Could you check a few things on this model? Use its own coordinates, in mm. A direction names the side the tool comes from. Coordinates: 2 decimals unless noted, no trailing zeros. Order: outer loops, then holes, each group sorted by start corner. A loop starts at its lowest first (then second) coordinate and runs counter-clockwise, first axis right, second up. Notation, with made-up numbers: M -8,87 L 43,87 A14 cw 43,92 Z; hole C 60.5,78.25 d9. An arc over 180 degrees is marked long. One line per question, with ' | ' between items. Start each with the question number.
from build123d import *

# Parameters (mm, degrees)
F1_DEPTH      = 25.4
F2_W          = 25.4
F2_H          = 15.875
F3_DEPTH      = 12.701
F3_DEPTH_BACK = 76.201
F5_DEPTH      = 9.525
F6_R          = 3.683
F7_DEPTH      = 82.551
F8_W          = 25.4
F8_H          = 12.7
F9_DEPTH      = 76.201
F10_R         = 3.683
F11_DEPTH     = 12.701
F12_R         = 8.89
F13_DEPTH     = 7.62


with BuildPart() as f1:
    # F0 (on Front) → F1 (new body, symmetric)
    with BuildSketch(Plane.XZ):
        Polygon((76.2, 0), (0, 0), (0, 63.5), (50.8, 63.5), (50.8, 73.025), (0, 82.55), (-12.7, 82.55), (-12.7, -82.55), (0, -82.55), (0, -31.75), (76.2, -19.05), align=None)
    extrude(amount=F1_DEPTH, both=True)

    # F2 (on Right) → F3 (cut, two sides)
    with BuildSketch(Plane.YZ) as f3_sk:
        with Locations((0, 74.6125)):
            Rectangle(F2_W, F2_H)
    extrude(amount=-F3_DEPTH, mode=Mode.SUBTRACT)
    extrude(f3_sk.sketch, amount=F3_DEPTH_BACK, mode=Mode.SUBTRACT)

    # F4 (on Top) → F5 (cut)
    with BuildSketch(Plane.XY):
        Polygon((19.304, -3.8128211777), (19.304, 3.8128211777), (12.7, 7.6256423555), (6.096, 3.8128211777), (6.096, -3.8128211777), (12.7, -7.6256423555), align=None)
        Polygon((70.1092849155, 3.8036527495), (63.5105825496, 7.6256350124), (56.901297634, 3.821982263), (56.8907150845, -3.8036527495), (63.4894174504, -7.6256350124), (70.098702366, -3.821982263), align=None)
    extrude(amount=-F5_DEPTH, mode=Mode.SUBTRACT)

    # F6 (on Top) → F7 (cut, through all)
    with BuildSketch(Plane.XY):
        with Locations((12.7, 0)):
            Circle(F6_R)
        with Locations((63.5, 0)):
            Circle(F6_R)
    extrude(amount=-F7_DEPTH, mode=Mode.SUBTRACT)

    # F8 (on Right) → F9 (cut, through all)
    with BuildSketch(Plane.YZ):
        with Locations((0, -25.4)):
            Rectangle(F8_W, F8_H)
    extrude(amount=F9_DEPTH, mode=Mode.SUBTRACT)

    # F10 (on Right) → F11 (cut, through all)
    with BuildSketch(Plane.YZ):
        with Locations((-12.7, -44.45)):
            Circle(F10_R)
        with Locations((12.7, -44.45)):
            Circle(F10_R)
        with Locations((-12.7, -69.85)):
            Circle(F10_R)
        with Locations((12.7, -69.85)):
            Circle(F10_R)
        with Locations((-12.7, 19.05)):
            Circle(F10_R)
        with Locations((12.7, 19.05)):
            Circle(F10_R)
        with Locations((-12.7, 44.45)):
            Circle(F10_R)
        with Locations((12.7, 44.45)):
            Circle(F10_R)
    extrude(amount=-F11_DEPTH, mode=Mode.SUBTRACT)

    # F12 (on Right) → F13 (cut)
    with BuildSketch(Plane.YZ):
        with Locations((-12.7, 44.45)):
            Circle(F12_R)
        with Locations((12.7, 44.45)):
            Circle(F12_R)
        with Locations((-12.7, 19.05)):
            Circle(F12_R)
        with Locations((12.7, 19.05)):
            Circle(F12_R)
    extrude(amount=-F13_DEPTH, mode=Mode.SUBTRACT)


solid = f1.part
(1) Imagine slicing it at B-B, the plane z = 44.45. Write out the boundary of the cut face in (x, y).
(2) Imagine slicing it at A-A, the plane z = -2.5. Write out the boundary of the cut face in (x, y), plus the area to 3 significant figures.
(3) Imagine slicing it at D-D, the plane y = 0. Write out the boundary of the cut face in (x, z) (3 decimals).
(4) We'd pull the mould along Z, two halves only. Please class faces 1 (the flat face through (37.57, -19.14, -25.49)), 2 (the flat face through (-6, -19, 82.55)), 3 (the flat face through (76.2, 0, -10)), 4 (the cylindrical face through (-10.124, 11.902, 15.455)): +Z half, -Z half, draft (parallel to the pull), parting line (faces both ways), or undercut.
(5) On a 3-axis mill with a long thin cutter (end or side, diameter ignored), from which of +Z, -Z, +X, -X, +Y, -Y can I reach the whole of each face in a straight line? I mean faces 5 (the flat face through (12, 12.7, 73)), 6 (the flat face through (0, 0, 31)), 7 (the cylindrical face through (-3.76, -4.22, 47.12)), 8 (the flat face through (66.75, -5.75, -4.7)). Say none if no direction works.
(6) If I drill on line 1 along Y through (x, z) = (-10, 19); line 2 along Z through (x, y) = (-10, -12) (3 decimals); line 3 along Y through (x, z) = (-5, 24.5), over which ranges is the centre line in solid material (lowest first)? Write a range as from..to.
(7) Imagine slicing it at C-C, the plane x = 28. Write out the boundary of the cut face in (y, z) (3 decimals), plus the area to 3 significant figures.
(8) For P1, Ø6.5, axis at x = 12.5, y = -2.5, coming from the +Z side (3 decimals); P2, Ø20.5, axis at x = 13, y = 5.5, coming from the +Z side; P3, Ø3, axis at x = 64, y = -13.5, coming from the -Z side, each with a flat end and sliding along its axis, tell me the tip position at first contact or that it passes through.
Answers:
1) outline: M -12.7,-25.4 L 0,-25.4 L 0,-21.59 L -7.62,-21.59 L -7.62,-16.38 L -12.7,-16.38 Z; M -12.7,-9.02 L -7.62,-9.02 L -7.62,-3.81 L 0,-3.81 L 0,3.81 L -7.62,3.81 L -7.62,9.02 L -12.7,9.02 Z; M -12.7,16.38 L -7.62,16.38 L -7.62,21.59 L 0,21.59 L 0,25.4 L -12.7,25.4 Z
2) outline: M -12.7,-25.4 L 76.2,-25.4 L 76.2,25.4 L -12.7,25.4 Z; hole M 6.1,-3.81 L 12.7,-7.63 L 19.3,-3.81 L 19.3,3.81 L 12.7,7.63 L 6.1,3.81 Z; hole M 56.89,-3.8 L 63.49,-7.63 L 70.1,-3.82 L 70.11,3.8 L 63.51,7.63 L 56.9,3.82 Z | area: 4,210 mm²
3) outline: M -12.7,-82.55 L 0,-82.55 L 0,-19.05 L 9.017,-19.05 L 9.017,-9.525 L 6.096,-9.525 L 6.096,0 L 0,0 L 0,63.5 L 50.8,63.5 L 50.8,66.675 L -12.7,66.675 Z; M 16.383,-19.05 L 59.817,-19.05 L 59.817,-9.525 L 56.896,-9.525 L 56.896,0 L 19.304,0 L 19.304,-9.525 L 16.383,-9.525 Z; M 67.183,-19.05 L 76.2,-19.05 L 76.2,0 L 70.104,0 L 70.104,-9.525 L 67.183,-9.525 Z
4) face 1: -Z half | face 2: +Z half | face 3: draft | face 4: undercut
5) face 5: +Z, +X, -X | face 6: +X, +Y, -Y | face 7: +X | face 8: +Z
6) line 1: -25.4..-16.38, -9.02..9.02, 16.38..25.4 | line 2: -82.55..-73.466, -66.234..-48.066, -40.834..15.434, 22.666..40.834, 48.066..66.675 | line 3: -25.4..-19.72, -5.68..5.68, 19.72..25.4
7) outline: M -25.4,-27.083 L -12.7,-27.083 L -12.7,-19.05 L 12.7,-19.05 L 12.7,-27.083 L 25.4,-27.083 L 25.4,0 L -25.4,0 Z; M -25.4,63.5 L 25.4,63.5 L 25.4,77.3 L 12.7,77.3 L 12.7,66.675 L -12.7,66.675 L -12.7,77.3 L -25.4,77.3 Z | area: 1,600 mm²
8) P1: z = 66.675 | P2: z = 81.48 | P3: z = -21.33
